from build123d import *

# Parameters (mm, degrees)
EXTRUDE_1_DEPTH     = 4
EXTRUDE_3_DEPTH     = 4
FILLET_1_R          = 10
FILLET_2_R          = 10
FILLET_3_R          = 10
FILLET_4_R          = 20
SKETCH_11_W         = 105
SKETCH_11_H         = 70
CUT_EXTRUDE_1_DEPTH = 10
FILLET_7_R          = 3
EXTRUDE_4_DEPTH     = 4
FILLET_8_R          = 30
SKETCH_13_R         = 1.75
CUT_EXTRUDE_2_DEPTH = 10
SKETCH_14_R         = 1.75
CUT_EXTRUDE_3_DEPTH = 10
SKETCH_15_R         = 2.75
CUT_EXTRUDE_4_DEPTH = 10
SKETCH_16_R         = 8.25
CUT_EXTRUDE_5_DEPTH = 10
SKETCH_18_R         = 1.75
CUT_EXTRUDE_6_DEPTH = 10


with BuildPart() as part:
    # ｽｹｯﾁ8 → ﾎﾞｽ - 押し出し1 (new body)
    with BuildSketch(Plane.XY):
        with BuildLine():
            Line((-110.970347899, 57.537656255), (-92.986343016, 83.537656255))
            Line((-92.986343016, 83.537656255), (-60.5, 105))
            Line((-60.5, 105), (60.5, 105))
            Line((60.5, 105), (92.986343016, 83.537656255))
            Line((92.986343016, 83.537656255), (110.970347899, 57.537656255))
            ThreePointArc((110.970347899, 57.537656255), (123.070502428, -21.878103945), (84.341344527, -92.257994794))
            Line((84.341344527, -92.257994794), (-84.341344527, -92.257994794))
            ThreePointArc((-84.341344527, -92.257994794), (-123.070502428, -21.878103945), (-110.970347899, 57.537656255))
        make_face()
        with BuildLine():
            Line((-89.302855497, 45), (-83.516465442, 55))
            Line((-83.516465442, 55), (-65, 48.260557735))
            Line((-65, 48.260557735), (-60, 15))
            Line((-60, 15), (-98.868599666, 15))
            ThreePointArc((-98.868599666, 15), (-95.273942579, 30.378872023), (-89.302855497, 45))
        make_face(mode=Mode.SUBTRACT)
        with BuildLine():
            Line((89.302855497, 45), (83.516465442, 55))
            Line((83.516465442, 55), (65, 48.260557735))
            Line((65, 48.260557735), (60, 15))
            Line((60, 15), (98.868599666, 15))
            ThreePointArc((98.868599666, 15), (95.273942579, 30.378872023), (89.302855497, 45))
        make_face(mode=Mode.SUBTRACT)
        with BuildLine():
            Line((-56.993435865, -5), (-48.304740393, -62.798171475))
            Line((-48.304740393, -62.798171475), (-73.194926437, -68.13591376))
            ThreePointArc((-73.194926437, -68.13591376), (-92.113131484, -38.9251976), (-99.874921777, -5))
            Line((-99.874921777, -5), (-56.993435865, -5))
        make_face(mode=Mode.SUBTRACT)
        with BuildLine():
            Line((56.993435865, -5), (48.304740393, -62.798171475))
            Line((48.304740393, -62.798171475), (73.194926437, -68.13591376))
            ThreePointArc((73.194926437, -68.13591376), (92.113131484, -38.9251976), (99.874921777, -5))
            Line((99.874921777, -5), (56.993435865, -5))
        make_face(mode=Mode.SUBTRACT)
    extrude(amount=-EXTRUDE_1_DEPTH)

    # ｽｹｯﾁ10 → ﾎﾞｽ - 押し出し3 (add)
    with BuildSketch(Plane.XY):
        Polygon((-99.874921777, -15), (-89.874921777, -5), (-99.874921777, -5), align=None)
        Polygon((-98.868599666, 15), (-88.868599666, 15), (-98.868599666, 25), align=None)
        Polygon((88.868599666, 15), (98.868599666, 15), (98.868599666, 25), align=None)
        Polygon((89.874921777, -5), (99.874921777, -5), (99.874921777, -15), align=None)
    extrude(amount=-EXTRUDE_3_DEPTH)

    # ﾌｨﾚｯﾄ1
    fillet_1_edges = [part.edges().sort_by_distance(p)[0] for p in [
        (-97.232371907, 23.363772241, -2),
        (-88.868599666, 15, -2),
        (88.868599666, 15, -2),
        (97.232371907, 23.363772241, -2),
        (98.997711183, -14.122789405, -2),
        (89.874921777, -5, -2),
        (-48.304740393, -62.798171475, -2),
        (-73.194926437, -68.13591376, -2),
        (48.304740393, -62.798171475, -2),
        (73.194926437, -68.13591376, -2),
        (-98.997711183, -14.122789405, -2),
        (-89.874921777, -5, -2),
    ]]
    fillet(fillet_1_edges, radius=FILLET_1_R)

    # ﾌｨﾚｯﾄ2
    fillet_2_edges = [part.edges().sort_by_distance(p)[0] for p in [
        (-56.993435865, -5, -2),
        (-60, 15, -2),
        (56.993435865, -5, -2),
        (60, 15, -2),
    ]]
    fillet(fillet_2_edges, radius=FILLET_2_R)

    # ﾌｨﾚｯﾄ3
    fillet_3_edges = [part.edges().sort_by_distance(p)[0] for p in [
        (-65, 48.260557735, -2),
        (-83.516465442, 55, -2),
        (83.516465442, 55, -2),
        (65, 48.260557735, -2),
    ]]
    fillet(fillet_3_edges, radius=FILLET_3_R)

    # ﾌｨﾚｯﾄ4
    fillet_4_edges = [part.edges().sort_by_distance(p)[0] for p in [
        (84.341344527, -92.257994794, -2),
        (-84.341344527, -92.257994794, -2),
    ]]
    fillet(fillet_4_edges, radius=FILLET_4_R)

    # ｽｹｯﾁ11 → ｶｯﾄ - 押し出し1 (cut)
    with BuildSketch(Plane.XY):
        with Locations((0, 63)):
            Rectangle(SKETCH_11_W, SKETCH_11_H)
    extrude(amount=-CUT_EXTRUDE_1_DEPTH, mode=Mode.SUBTRACT)

    # ﾌｨﾚｯﾄ7
    fillet_7_edges = [part.edges().sort_by_distance(p)[0] for p in [
        (52.5, 98, -2),
        (52.5, 28, -2),
        (-52.5, 28, -2),
        (-52.5, 98, -2),
    ]]
    fillet(fillet_7_edges, radius=FILLET_7_R)

    # ｽｹｯﾁ12 → ﾎﾞｽ - 押し出し4 (add)
    with BuildSketch(Plane.XY):
        with BuildLine():
            add(Edge.make_bspline(
                [(-92.986343016, 83.537656255), (-79.595640691, 97.18270504), (-60.5, 105)],
                knots=[0.448106601, 0.448106601, 0.448106601, 1, 1, 1], degree=2))
            Line((-92.986343016, 83.537656255), (-60.5, 105))
        make_face()
        with BuildLine():
            add(Edge.make_bspline(
                [(-110.970347899, 57.537656255), (-103.858845057, 72.4586391), (-92.986343016, 83.537656255)],
                knots=[0, 0, 0, 0.448106601, 0.448106601, 0.448106601], degree=2))
            Line((-110.970347899, 57.537656255), (-92.986343016, 83.537656255))
        make_face()
        with BuildLine():
            add(Edge.make_bspline(
                [(92.986343016, 83.537656255), (79.595640691, 97.18270504), (60.5, 105)],
                knots=[0.448106601, 0.448106601, 0.448106601, 1, 1, 1], degree=2))
            Line((60.5, 105), (92.986343016, 83.537656255))
        make_face()
        with BuildLine():
            add(Edge.make_bspline(
                [(110.970347899, 57.537656255), (103.858845057, 72.4586391), (92.986343016, 83.537656255)],
                knots=[0, 0, 0, 0.448106601, 0.448106601, 0.448106601], degree=2))
            Line((92.986343016, 83.537656255), (110.970347899, 57.537656255))
        make_face()
    extrude(amount=-EXTRUDE_4_DEPTH)

    # ﾌｨﾚｯﾄ8
    fillet_8_edges = [part.edges().sort_by_distance(p)[0] for p in [
        (-60.5, 105, -2),
        (60.5, 105, -2),
    ]]
    fillet(fillet_8_edges, radius=FILLET_8_R)

    # ｽｹｯﾁ13 → ｶｯﾄ - 押し出し2 (cut)
    with BuildSketch(Plane.XY):
        with Locations((107, 35)):
            Circle(SKETCH_13_R)
        with Locations((113, 5)):
            Circle(SKETCH_13_R)
        with Locations((78, 5)):
            Circle(SKETCH_13_R)
        with Locations((101, -50)):
            Circle(SKETCH_13_R)
        with Locations((-101, -50)):
            Circle(SKETCH_13_R)
        with Locations((-78, 5)):
            Circle(SKETCH_13_R)
        with Locations((-113, 5)):
            Circle(SKETCH_13_R)
        with Locations((-107, 35)):
            Circle(SKETCH_13_R)
    extrude(amount=-CUT_EXTRUDE_2_DEPTH, mode=Mode.SUBTRACT)

    # ｽｹｯﾁ14 → ｶｯﾄ - 押し出し3 (cut)
    with BuildSketch(Plane.XY):
        with Locations((-65, 90)):
            Circle(SKETCH_14_R)
        with Locations((-55, 20)):
            Circle(SKETCH_14_R)
        with Locations((-49.738512764, -15)):
            Circle(SKETCH_14_R)
        with Locations((-39.627739016, -82.257994794)):
            Circle(SKETCH_14_R)
        with Locations((65, 90)):
            Circle(SKETCH_14_R)
        with Locations((55, 20)):
            Circle(SKETCH_14_R)
        with Locations((49.738512764, -15)):
            Circle(SKETCH_14_R)
        with Locations((39.627739016, -82.257994794)):
            Circle(SKETCH_14_R)
    extrude(amount=-CUT_EXTRUDE_3_DEPTH, mode=Mode.SUBTRACT)

    # ｽｹｯﾁ15 → ｶｯﾄ - 押し出し4 (cut)
    with BuildSketch(Plane.XY):
        with Locations((-21.650635095, 12.5)):
            Circle(SKETCH_15_R)
        with Locations((21.650635095, 12.5)):
            Circle(SKETCH_15_R)
        with Locations((0, -25)):
            Circle(SKETCH_15_R)
    extrude(amount=-CUT_EXTRUDE_4_DEPTH, mode=Mode.SUBTRACT)

    # ｽｹｯﾁ16 → ｶｯﾄ - 押し出し5 (cut)
    with BuildSketch(Plane.XY):
        with Locations((84, 68)):
            Circle(SKETCH_16_R)
    extrude(amount=-CUT_EXTRUDE_5_DEPTH, mode=Mode.SUBTRACT)

    # ｽｹｯﾁ18 → ｶｯﾄ - 押し出し6 (cut)
    with BuildSketch(Plane.XY):
        with Locations((-42, 5)):
            Circle(SKETCH_18_R)
        with Locations((42, 5)):
            Circle(SKETCH_18_R)
    extrude(amount=-CUT_EXTRUDE_6_DEPTH, mode=Mode.SUBTRACT)


solid = part.part
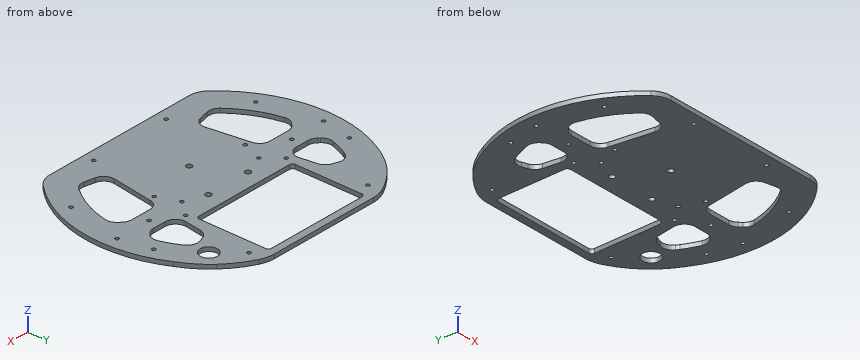
Here's how the part is built. I have some questions about the finished solid (model axes, mm). Give positions to 0.01 mm unless a question says otherwise; leave off trailing zeros. Order: outer loops, then holes, each group sorted by start corner. A loop starts at its lowest first (then second) coordinate and runs counter-clockwise, first axis right, second up. Notation, with made-up numbers: (4.25, 37.5) -> (28.25, 37.5) arc R23 ccw to (28.25, 63.5) -> close; hole circle Ø7 at (27, 9). An arc over 180 degrees is marked (long way). Use a Markdown table: item, result. Add a question column.
Item 1: I need wall thicknesses on line 1 (X direction, y = 43.5, z = -2.9); line 2 (Y direction, x = 83, z = -2.85); line 3 (Y direction, x = -33, z = -1.25). Which ranges of each line are inside material? Lowest first, please.
Item 2: Imagine slicing it at D-D on y = -76.5. Please give me the cut outline in (x, z).
Item 3: Imagine slicing it at A-A on y = -25. Please give me the cut outline in (x, z), plus the area to 3 significant figures.
Item 4: Imagine slicing it at B-B on y = 68. Give the number of separate pieces and of enclosed holes in the cut face, plus the area to 3 significant figures.
Item 5: Will these pins go through, and if not, where does the flat tip stop? pin 1 (2 mm diameter, centred on x = 42, y = 5, fed in from +Z); pin 2 (1.2 mm diameter, centred on x = -75.5, z = -3, fed in from +Y); pin 3 (2 mm diameter, centred on y = 62.5, z = -1.5, fed in from -X).
Data:
| question | item | result |
|---|---|---|
| 1 | line 1 | x = -117.19 to -90.04, -64.35 to -52.5, 52.5 to 64.35, 90.04 to 117.19 |
| 1 | line 2 | y = -91.06 to -55.78, -5 to 15, 51.93 to 59.81, 76.19 to 92.31 |
| 1 | line 3 | y = -92.26 to 28, 98 to 105 |
| 2 | outline | (-98.86, -4) -> (98.86, -4) -> (98.86, 0) -> (-98.86, 0) -> close |
| 3 | outline | (-122.47, -4) -> (-96.82, -4) -> (-96.82, 0) -> (-122.47, 0) -> close; (-53.99, -4) -> (-2.75, -4) -> (-2.75, 0) -> (-53.99, 0) -> close; (2.75, -4) -> (53.99, -4) -> (53.99, 0) -> (2.75, 0) -> close; (96.82, -4) -> (122.47, -4) -> (122.47, 0) -> (96.82, 0) -> close |
| 3 | area | 615 mm² |
| 4 | separate pieces | 3 |
| 4 | enclosed holes | 0 |
| 4 | area | 356 mm² |
| 5 | pin 1 | passes through |
| 5 | pin 2 | stops at y = 97.79 |
| 5 | pin 3 | stops at x = -108.98 |
